Autodesk Inventor part; units mm, degrees
ref_plane "YZ Plane" through (0, 0, 0) normal (1, 0, 0) x (0, 1, 0)
ref_plane "XZ Plane" through (0, 0, 0) normal (0, 1, 0) x (-1, 0, 0)
ref_plane "XY Plane" through (0, 0, 0) normal (0, 0, 1) x (1, 0, 0)
sketch "Sketch1" plane through (0, 0, 0) normal (0, 1, 0) x (-1, 0, 0)
  line L0 (7.75, -19.9274) -> (7.75, -42.3236) construction
  line L1 (13.2323, -27.5) -> (6.4845, -27.5) construction
  line L2 (15.5, -10) -> (17.95, -10)
  line L3 (17.95, -10) -> (17.95, -20)
  line L4 (17.95, -20) -> (15.5, -20)
  line L5 (15.5, -35) -> (17.95, -35)
  line L6 (17.95, -35) -> (17.95, -45)
  line L7 (17.95, -45) -> (15.5, -45)
  line L8 (0, -10) -> (-2.45, -10)
  line L9 (-2.45, -10) -> (-2.45, -20)
  line L10 (-2.45, -20) -> (0, -20)
  line L11 (0, -35) -> (-2.45, -35)
  line L12 (-2.45, -45) -> (0, -45)
  line L13 (-2.45, -45) -> (-2.45, -35)
  line L14 (15.5, -10) -> (15.5, 0)
  line L15 (15.5, -55) -> (15.5, -45)
  line L16 (15.5, -35) -> (15.5, -20)
  line L17 (0, 0) -> (0, -10)
  line L18 (0, -20) -> (0, -35)
  line L19 (0, -45) -> (0, -55)
  line L20 (4.25, 0) -> (0, 0)
  line L21 (0, -55) -> (4.25, -55)
  line L22 (11.25, -55) -> (15.5, -55)
  line L23 (4.25, 0) -> (4.25, 2.45)
  line L24 (4.25, 2.45) -> (11.25, 2.45)
  line L25 (11.25, 2.45) -> (11.25, 0)
  line L26 (11.25, 0) -> (15.5, 0)
  line L27 (11.25, -55) -> (11.25, -57.45)
  line L28 (11.25, -57.45) -> (4.25, -57.45)
  line L29 (4.25, -57.45) -> (4.25, -55)
  line L30 (5, -35) -> (3, -35)
  line L31 (3, -35) -> (3, -20)
  line L32 (3, -20) -> (5, -20)
  line L33 (5, -20) -> (5, -35)
  dimension "d8" = 10
  dimension "d9" = 15
  dimension "d10" = 15.5
  dimension "d17" = 2.45
  dimension "d19" = 7
  dimension "d20" = 55
  dimension "d21" = 3
  dimension "d22" = 15
  dimension "d23" = 2
extrude "Extrusion1" add sketch "Sketch1" along normal blind 3
properties part number "Front_wall"
The listing builds one solid part. Answer for the finished solid, in the listing's coordinates (mm). A direction names the side the tool comes from. Round coordinates to 2 decimals unless told otherwise and drop trailing zeros. Write each loop counter-clockwise with the first axis right and the second up, starting at its lowest first coordinate (ties: lowest second). Pieces come first, ordered by that corner, then holes. Notation, with made-up numbers: (72.5, 81) - (97.5, 81) arc R33 cw to (97.5, 113) - close; hole circle Ø3 at (-33, 11). An arc over 180 degrees is marked (long way). Use one line per item in the form item = value. Start each with the question number.
Item 1: A cutting plane is placed at D-D (z = -46.5). Write down the section's boundary in (x, y), plus the area to 3 significant figures.
Item 2: A tool of negligible diameter and unlimited length cuts with its end or side. For faces 1 (the flat face through (1, 1, -35)), 2 (the flat face through (-13, 1, 0)), 3 (the flat face through (-3, 1, -28)), 4 (the flat face through (-4.25, 1, -56)), 5 (the flat face through (-11.25, 1, -56)), from which of +Z, -Z, +X, -X, +Y, -Y can it reach the whole face along a straight path? Write none if from no direction.
Item 3: Determine the mould class of faces 6 (the flat face through (-4, 1, -20)), 7 (the flat face through (1, 1, -10)), 8 (the flat face through (2.45, 1, -15)), 9 (the flat face through (-5, 1, -27)) for opening direction X: +X half, -X half, draft (parallel to the pull), parting line (faces both ways), or undercut.
Item 4: Find the intervals of material crossed by line 1 (X direction, y = 0.45, z = -32.5); line 2 (Z direction, x = -16, y = 0.2); line 3 (X direction, y = 1.3, z = -9.5), in increasing order. Write a range as [from, to].
Item 5: Flat-ended cylindrical pins translate along their axes: pin 1 Ø1.5 at (y, z) = (1, -24) entering from +X; pin 2 Ø1.2 at (x, y) = (-17, 1) entering from +Z; pin 3 Ø0.6 at (x, y) = (-3.5, 1.5) entering from -Z. Find the tip coordinate at first contact, or state that the pin passes through.
Item 6: A cutting plane is placed at A-A (z = -24). Write down the section's boundary in (x, y), plus the area to 3 significant figures.
Item 7: A cutting plane is placed at C-C (x = -14). Write down the section's boundary in (y, z).
The answers:
q1.outline = (-15.5, 0) - (0, 0) - (0, 3) - (-15.5, 3) - close
q1.area = 46.5 mm^2
q2.face_1 = +X, +Y, -Y
q2.face_2 = +Z, -X, +Y, -Y
q2.face_3 = +Y, -Y
q2.face_4 = -Z, +X, +Y, -Y
q2.face_5 = -Z, -X, +Y, -Y
q3.face_6 = undercut
q3.face_7 = draft
q3.face_8 = +X half
q3.face_9 = undercut
q4.line_1 = [-15.5, -5], [-3, 0]
q4.line_2 = [-45, -35], [-20, -10]
q4.line_3 = [-15.5, 0]
q5.pin_1 = 0
q5.pin_2 = -10
q5.pin_3 = -55
q6.outline = (-15.5, 0) - (-5, 0) - (-5, 3) - (-15.5, 3) - close; (-3, 0) - (0, 0) - (0, 3) - (-3, 3) - close
q6.area = 40.5 mm^2
q7.outline = (0, -55) - (3, -55) - (3, 0) - (0, 0) - close
